Could you check a few things on this model? Use its own coordinates, in mm. A direction names the side the tool comes from. Give positions to 0.01 mm unless a question says otherwise; leave off trailing zeros. Loops run counter-clockwise (first coordinate to the right, second up) from the corner with the lowest first, then second, coordinate; pieces in that order, holes last. Notation, with made-up numbers: M 53,89 L 99,89 A33 cw 99,127 Z; hole C 78,-35 d5. An arc over 180 degrees is marked long. Answer in a Markdown table with one row per item. Add a question column.
1. Thinking about a two-plate mould opening in Y: for faces 1 (the flat face through (0, 0, 76.2)), 2 (the cylindrical face through (-1.38, -6.2, 21.91)), 3 (the flat face through (76.2, 0, 60)), 4 (the flat face through (-76.2, 0, 60)), which applies, released by +Y, released by -Y, zero draft, split by the parting line, or undercut?
2. I need wall thicknesses on line 1 along Z through (x, y) = (4.5, -10); line 2 along X through (y, z) = (-8, 63); line 3 along Z through (x, y) = (18.5, 0). Which ranges of each line are inside material? Lowest first, please. Write a range as from..to.
3. If we section it at D-D on y = -12.5: List the corners of the cut face in (x, z) for me, then the cut area to 3 significant figures.
4. I'm going to push flat-ended pins straight in: pin 1 Ø10 at (y, z) = (-9, 64) entering from -X; pin 2 Ø6 at (y, z) = (2.5, 20) entering from +X; pin 3 Ø7 at (y, z) = (-2, 59.5) entering from +X. Where does each tip first touch, or does it pass through?
5. If we section it at C-C on y = 8.5: List the corners of the cut face in (x, z) for me (3 decimals), then the cut area to 3 significant figures.
6. If we section it at A-A on x = 0: List the corners of the cut face in (y, z) for me (3 decimals).
7. Which directions (+Z, -Z, +X, -X, +Y, -Y) give clear straight access to the entire face, cutting with the end or side of a thin tool? Please do faces 5 (the flat face through (7, 0, 44.45)), 6 (the flat face through (0, 0, 0)).
8. If we section it at B-B on z = 23.5: List the corners of the cut face in (x, y) for me.
```python
from build123d import *

# Parameters (mm, degrees)
F0_R     = 6.35
F1_DEPTH = 76.2
F2_R     = 15.875
F3_DEPTH = 31.75
F5_DEPTH = 76.2


with BuildPart() as f1:
    # F0 (on Top) → F1 (new body)
    with BuildSketch(Plane.XY):
        Circle(F0_R)
    extrude(amount=F1_DEPTH)

    # F2 (on face) → F3 (join)
    with BuildSketch(Plane.XY.offset(76.2)):
        Circle(F2_R)
    extrude(amount=-F3_DEPTH)

    # F4 (on Right) → F5 (join, symmetric)
    with BuildSketch(Plane.YZ):
        with BuildLine():
            ThreePointArc((0, 55.88), (3.1430896424, 57.1819103576), (4.445, 60.325))
            ThreePointArc((4.445, 60.325), (-3.1430896424, 63.4680896424), (0, 55.88))
        make_face()
    extrude(amount=F5_DEPTH, both=True)

    # F6 (on face) → F7 (revolve)
    with BuildSketch(Plane.YZ.offset(76.2)):
        with BuildLine():
            Line((4.445, 60.325), (10.16, 60.325))
            ThreePointArc((10.16, 60.325), (0, 70.485), (-10.16, 60.325))
            Line((-10.16, 60.325), (-4.445, 60.325))
            ThreePointArc((-4.445, 60.325), (0, 64.77), (4.445, 60.325))
        make_face()
    revolve(axis=Axis((76.2, -5.08, 60.325), (0, -1, 0)))

    # F8 (on face) → F9 (revolve)
    with BuildSketch(Plane(origin=(-76.2, 0, 0), x_dir=(0, -1, 0), z_dir=(-1, 0, 0))):
        with BuildLine():
            Line((4.445, 60.325), (10.16, 60.325))
            ThreePointArc((10.16, 60.325), (0, 70.485), (-10.16, 60.325))
            Line((-10.16, 60.325), (-4.445, 60.325))
            ThreePointArc((-4.445, 60.325), (0, 64.77), (4.445, 60.325))
        make_face()
    revolve(axis=Axis((-76.2, 0, 60.325), (0, -1, 0)))


solid = f1.part
```
Results:
| question | item | result |
|---|---|---|
| 1 | face 1 | zero draft |
| 1 | face 2 | split by the parting line |
| 1 | face 3 | undercut |
| 1 | face 4 | undercut |
| 2 | line 1 | 44.45..76.2 |
| 2 | line 2 | -81.86..-70.54, -13.71..13.71, 70.54..81.86 |
| 2 | line 3 | 55.88..64.77 |
| 3 | outline | M -9.79,44.45 L 9.79,44.45 L 9.79,76.2 L -9.79,76.2 Z |
| 3 | area | 621 mm2 |
| 4 | pin 1 | x = -85.2 |
| 4 | pin 2 | x = 6.35 |
| 4 | pin 3 | x = 86.36 |
| 5 | outline | C -76.2,60.325 d11.131; M -13.408,44.45 L 13.408,44.45 L 13.408,76.2 L -13.408,76.2 Z; C 76.2,60.325 d11.131 |
| 5 | area | 1,050 mm2 |
| 6 | outline | M -15.875,44.45 L -6.35,44.45 L -6.35,0 L 6.35,0 L 6.35,44.45 L 15.875,44.45 L 15.875,76.2 L -15.875,76.2 Z |
| 7 | face 5 | -Z |
| 7 | face 6 | -Z, +X, -X, +Y, -Y |
| 8 | outline | C 0,0 d12.7 |
